```python
from build123d import *

# Parameters (mm, degrees)
SKETCH1_W           = 94
SKETCH1_H           = 8.9
BOSS_EXTRUDE1_DEPTH = 6
BOSS_EXTRUDE2_DEPTH = 10
FILLET1_R           = 1


with BuildPart() as part:
    # Sketch1 → Boss-Extrude1 (new body)
    with BuildSketch(Plane(origin=(0, 0, 0), x_dir=(1, 0, 0), z_dir=(0, 1, 0))):
        Polygon((106.5, 2.9), (106.5, 5.15), (108.9, 5.15), (108.9, -2.25), (106.5, -2.25), (106.5, 0), (81.5, 0), (81.5, -6), (-18.5, -6), (-18.5, -0.05), (-48.5, -0.05), (-48.5, -6), (-68.5, -6), (-68.5, 0), (-108.8, 0), (-108.8, -2.25), (-111.2, -2.25), (-111.2, 5.15), (-108.8, 5.15), (-108.8, 2.9), (-68.5, 2.9), (-68.5, 8.9), (-48.5, 8.9), (-48.5, 2.95), (-18.5, 2.95), (-18.5, 8.9), (81.5, 8.9), (81.5, 2.9), align=None)
        with Locations((31.5, 1.45)):
            Rectangle(SKETCH1_W, SKETCH1_H, mode=Mode.SUBTRACT)
    extrude(amount=BOSS_EXTRUDE1_DEPTH)

    # Sketch2 → Boss-Extrude2 (add)
    with BuildSketch(Plane(origin=(0, 6, 0), x_dir=(1, 0, 0), z_dir=(0, 1, 0))):
        Polygon((-65.9, 6.9), (-65.9, 15.9), (-63.9, 15.9), (-63.9, 8.9), (-56.9, 8.9), (-56.9, 6.9), align=None)
        Polygon((-65.9, -4), (-56.9, -4), (-56.9, -6), (-63.9, -6), (-63.9, -13), (-65.9, -13), align=None)
        Polygon((65.9, -13), (65.9, -4), (56.9, -4), (56.9, -6), (63.9, -6), (63.9, -13), align=None)
        Polygon((56.9, 6.9), (65.9, 6.9), (65.9, 15.9), (63.9, 15.9), (63.9, 8.9), (56.9, 8.9), align=None)
    extrude(amount=-BOSS_EXTRUDE2_DEPTH)

    # Fillet1
    fillet1_edges = [part.edges().sort_by_distance(p)[0] for p in [
        (-68.5, 0, 3),
        (-68.5, 0, -5.9),
        (-108.8, 0, -4.025),
        (-108.8, 0, 1.125),
        (-68.5, 3, 0),
        (-68.5, 3, -2.9),
        (-88.65, 0, 0),
        (-88.65, 0, -2.9),
        (81.5, 0, -5.9),
        (81.5, 0, 3),
        (78.5, 3, -5.9),
        (78.5, 3, 3),
        (-15.5, 3, 3),
        (-15.5, 3, -5.9),
        (-18.5, 3, -2.95),
        (-18.5, 3, 0.05),
        (-48.5, 3, -2.95),
        (-48.5, 3, 0.05),
        (-65.9, 3, 6),
        (-65.9, 3, -8.9),
        (65.9, 3, -8.9),
        (65.9, 3, 6),
        (81.5, 3, -2.9),
        (81.5, 3, 0),
        (106.5, 0, 1.125),
        (107.7, 0, 2.25),
        (108.9, 0, -1.45),
        (107.7, 0, -5.15),
        (106.5, 0, -4.025),
        (94, 0, -2.9),
        (94, 0, 0),
    ]]
    fillet(fillet1_edges, radius=FILLET1_R)


solid = part.part
```
Could you check a few things on this model? Use its own coordinates, in mm. A direction names the side the tool comes from. Round coordinates to 2 decimals unless told otherwise and drop trailing zeros. Write each loop counter-clockwise with the first axis right and the second up, starting at its lowest first coordinate (ties: lowest second). Pieces come first, ordered by that corner, then holes. Notation, with made-up numbers: M 54,52 L 73,52 A21 cw 73,78 Z; hole C 56,80.5 d3. An arc over 180 degrees is marked long. Write each question's results on one line, items separated by ' | '. Start each with the question number.
1. Imagine slicing it at D-D on x = -62. List the corners of the cut face in (y, z) for me, and give its area (3 significant figures).
2. I need wall thicknesses on L1, parallel to Z at x = 46.5, y = 4.75; L2, parallel to X at y = 4.75, z = -7.5; L3, parallel to X at y = 4.25, z = -2.5. Which ranges of each line are inside material? Lowest first, please. Write a range as from..to.
3. Thinking about a two-plate mould opening in Z: for faces 1 (the face through (74, 3, -8.9)), 2 (the face through (-61, -2, 4)), 3 (the face through (74, 3, 6)), 4 (the face through (-15.5, 3, -1)), which applies, +Z half, -Z half, draft (parallel to the pull), parting line (faces both ways), or undercut?
4. I'm going to push flat-ended pins straight in: pin 1 Ø5 at (x, y) = (42, 0) entering from +Z; pin 2 Ø1.2 at (x, y) = (108, 3.5) entering from -Z; pin 3 Ø2.5 at (y, z) = (3, 4) entering from -X; pin 4 Ø1 at (x, z) = (34.5, -11) entering from -Y. Where does each tip first touch, or does it pass through?
5. On a 3-axis mill with a long thin cutter (end or side, diameter ignored), from which of +Z, -Z, +X, -X, +Y, -Y can I reach the whole of each face in a straight line? I mean faces 5 (the face through (22, 3, -8.9)), 6 (the face through (31, 3, -5.9)), 7 (the face through (-89, 3, 0)). Say none if no direction works.
6. Imagine slicing it at B-B on z = -12. List the corners of the cut face in (x, y) for me, and give its area (3 significant figures).
7. Imagine slicing it at C-C on x = 14. List the corners of the cut face in (y, z) for me, and give its area (3 significant figures).
8. Imagine slicing it at A-A on x = 60. List the corners of the cut face in (y, z) for me.
Result sheet:
1) outline: M -4,-8.9 L 6,-8.9 L 6,6 L -4,6 L -4,4 L 0,4 L 0,-6.9 L -4,-6.9 Z | area: 105 mm^2
2) L1: z = -8.9..-5.9, 3..6 | L2: x = -68.5..-48.5, -18.5..81.5 | L3: x = -111.2..-15.5, 78.5..108.9
3) face 1: -Z half | face 2: undercut | face 3: +Z half | face 4: undercut
4) pin 1: stops at z = 6 | pin 2: stops at z = -5.15 | pin 3: stops at x = -68.5 | pin 4: passes through
5) face 5: -Z, +Y, -Y | face 6: +Y, -Y | face 7: +Z, +Y, -Y
6) outline: M -65.9,-4 L -63.9,-4 L -63.9,6 L -65.9,6 Z; M 63.9,-4 L 65.9,-4 L 65.9,6 L 63.9,6 Z | area: 40.0 mm^2
7) outline: M 0,-8.9 L 6,-8.9 L 6,-5.9 L 0,-5.9 Z; M 0,3 L 6,3 L 6,6 L 0,6 Z | area: 36.0 mm^2
8) outline: M -4,-8.9 L 6,-8.9 L 6,-5.9 L 0,-5.9 L 0,-6.9 L -4,-6.9 Z; M -4,4 L 0,4 L 0,3 L 6,3 L 6,6 L -4,6 Z
